```python
from build123d import *

# Parameters (mm, degrees)
BOSS_EXTRUDE1_DEPTH = 2


with BuildPart() as part:
    # Sketch1 → Boss-Extrude1 (new body)
    with BuildSketch(Plane.XY):
        with BuildLine():
            Line((5, 7.5), (-15, 7.5))
            ThreePointArc((-15, 7.5), (-22.5, 0), (-15, -7.5))
            Line((-15, -7.5), (5, -7.5))
            Line((5, -7.5), (5, 7.5))
        make_face()
        with BuildLine():
            ThreePointArc((-12.450490243, -2.75), (-18.75, 0), (-12.450490243, 2.75))
            Line((-12.450490243, 2.75), (0, 2.25))
            ThreePointArc((0, 2.25), (1.590990258, 1.590990258), (2.25, 0))
            ThreePointArc((2.25, 0), (1.590990258, -1.590990258), (0, -2.25))
            Line((0, -2.25), (-12.450490243, -2.75))
        make_face(mode=Mode.SUBTRACT)
    extrude(amount=BOSS_EXTRUDE1_DEPTH)


solid = part.part
```
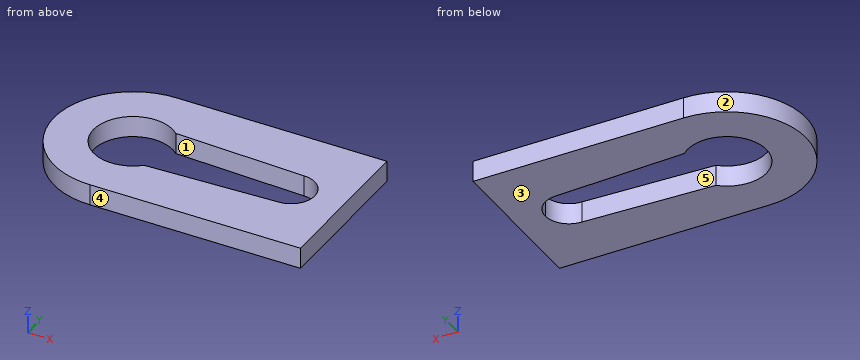
Input: part model. Units: mm. Frame: model coordinates. Face numbers are marked on the shaded views. A direction names the side the tool comes from. Coordinates: 2 decimals unless noted, no trailing zeros. Loops run counter-clockwise (first coordinate to the right, second up) from the corner with the lowest first, then second, coordinate; pieces in that order, holes last. Notation, with made-up numbers: M 11.25,26.25 L 56.25,26.25 A26 cw 56.25,55.25 Z; hole C 2.25,-30.75 d9. An arc over 180 degrees is marked long. Answer in a Markdown table with one row per item.
1. Material intervals for line 1 (Y direction, x = -15, z = 1.3); line 2 (Y direction, x = -18.25, z = 1.35); line 3 (X direction, y = 3, z = 1.3), sorted ascending.
Response:
| item | result |
|---|---|
| line 1 | y = -7.5 to -3.75, 3.75 to 7.5 |
| line 2 | y = -6.76 to -1.87, 1.87 to 6.76 |
| line 3 | x = -21.87 to -17.25, -12.75 to 5 |
2. Section C-C, the plane z = 1.6. Output: boundary loops of the cut face in (x, y), then the cut area to 3 significant figures.
Response:
| item | result |
|---|---|
| outline | M -15,-7.5 L 5,-7.5 L 5,7.5 L -15,7.5 A7.5 ccw Z; hole M -12.45,-2.75 L 0,-2.25 A2.25 ccw 0,2.25 L -12.45,2.75 A3.75 ccw long Z |
| area | 279 mm2 |
3. Section B-B, the plane x = -17.75. Output: boundary loops of the cut face in (y, z).
Response:
| item | result |
|---|---|
| outline | M -6.98,0 L -2.55,0 L -2.55,2 L -6.98,2 Z; M 2.55,0 L 6.98,0 L 6.98,2 L 2.55,2 Z |
4. Draft query along Y for the marked faces 1, 2 and 3. Return one class per face: pulls with the +Y half, pulls with the -Y half, needs draft (parallel to the pull), parting line crosses it, or undercut.
Response:
| item | result |
|---|---|
| face 1 | undercut |
| face 2 | parting line crosses it |
| face 3 | needs draft |
5. Section A-A, the plane y = 1.75. Output: boundary loops of the cut face in (x, z).
Response:
| item | result |
|---|---|
| outline | M -22.29,0 L -18.32,0 L -18.32,2 L -22.29,2 Z; M 1.41,0 L 5,0 L 5,2 L 1.41,2 Z |
6. Reachability of the marked faces 4 and 5 from +Z, -Z, +X, -X, +Y, -Y: full face, straight path, thin tool, end or side. Return the list, or none.
Response:
| item | result |
|---|---|
| face 4 | +Z, -Z, +X, -X, -Y |
| face 5 | +Z, -Z |
